from build123d import *

# Parameters (mm, degrees)
F0_W      = 19.9827682227
F0_H      = 13.8834062964
F2_R      = 5
F3_SIZE   = 5
F5_D      = 3
F7_D      = 3
F9_D      = 3
F11_DEPTH = 2


with BuildPart() as f1:
    # F0 (on Front) → F1 (revolve)
    with BuildSketch(Plane.XZ):
        Polygon((-5.1426226273, 40.0602705777), (-45.9897518158, 40.0602705777), (-45.9897518158, 11.2985512242), (-5.1426226273, 11.2985512242), (-5.1426226273, 26.1768642813), align=None)
        with Locations((4.848761484, 33.1185674295)):
            Rectangle(F0_W, F0_H)
    revolve(axis=Axis((-8.3751268685, 0, 0), (1, 0, 0)))

    # F2
    f2_edges = [f1.edges().sort_by_distance(p)[0] for p in [
        (14.840146, 0, -26.176864),
    ]]
    fillet(f2_edges, radius=F2_R)

    # F3
    f3_edges = [f1.edges().sort_by_distance(p)[0] for p in [
        (-5.142623, 0, -26.176864),
        (14.840146, 0, -40.060271),
        (-45.989752, 0, -40.060271),
        (-15.574803, 0, 40.060271),
    ]]
    chamfer(f3_edges, length=F3_SIZE)

    # F5 (through all)
    with Locations(Plane.YZ.offset(-5.1426226273)):
        with Locations((-16.2885512242, 0)):
            Hole(F5_D / 2)

    # F7 (through all)
    with Locations(Plane.YZ.offset(-5.1426226273)):
        with Locations((15.9020125866, 0)):
            Hole(F7_D / 2)

    # F9 (through all)
    with Locations(Plane.YZ.offset(-5.1426226273)):
        with Locations((0, 16.050176695)):
            Hole(F9_D / 2)

    # F10 (on face) → F11 (cut)
    with BuildSketch(Plane.YZ.offset(-5.1426226273)):
        with BuildLine():
            Line((5.9653543867, 17.550176695), (0, 17.550176695))
            ThreePointArc((0, 17.550176695), (1.0606601718, 17.1108368668), (1.5, 16.050176695))
            ThreePointArc((1.5, 16.050176695), (1.2449620199, 15.2134750941), (0.5665739081, 14.6612944081))
            Line((0.5665739081, 14.6612944081), (5.9653543867, 14.6612944081))
            Line((5.9653543867, 14.6612944081), (5.9653543867, 17.550176695))
        make_face()
    extrude(amount=-F11_DEPTH, mode=Mode.SUBTRACT)


solid = f1.part
Build history of the part. All positions in model axes, mm. A direction names the side the tool comes from. Round coordinates to 2 decimals unless told otherwise and drop trailing zeros. Write each loop counter-clockwise with the first axis right and the second up, starting at its lowest first coordinate (ties: lowest second). Pieces come first, ordered by that corner, then holes. Notation, with made-up numbers: M -35.5,6.5 L 21.5,6.5 A33 cw 21.5,34.5 Z; hole C 50.25,62 d5. An arc over 180 degrees is marked long. Use CSV: the item, a comma, the result in double quotes.
1. Two-plate mould, pull along Y, no slides. Class faces 1 (the face through (-25.85, -17.72, 0.45)), 2 (the face through (-6, 3, 14.661)), 3 (the face through (-45.747, 21.481, -28.015)), 4 (the face through (-45.99, -8.3, -8.3)): +Y half, -Y half, draft (parallel to the pull), parting line (faces both ways), or undercut.
Reply:
face 1,"undercut"
face 2,"undercut"
face 3,"parting line"
face 4,"draft"
2. Saw through at B-B (x = -33). Give the cut face in (y, z), plus the area to 3 significant figures.
Reply:
outline,"C 0,0 d80.12; hole C -16.29,0 d3; hole C 0,0 d22.6; hole C 0,16.05 d3; hole C 15.9,0 d3"
area,"4,620 mm²"
3. Wall check: probe 1 along Z at (x, y) = (-36, 0); probe 2 along Z at (x, y) = (-42, -10); probe 3 along Z at (x, y) = (-35, -16). Give the ranges that are in metal, low to high. Write a range as from..to.
Reply:
probe 1,"z = -40.06..-11.3, 11.3..14.55, 17.55..40.06"
probe 2,"z = -37.75..-5.26, 5.26..37.75"
probe 3,"z = -36.73..-1.47, 1.47..36.73"
4. Tool access for faces 5 (the face through (-25.28, 6.87, -8.97)), 6 (the face through (-6, 5.965, 16)): list every direction of +Z, -Z, +X, -X, +Y, -Y with a clear straight run to the whole face (end or side of a thin tool).
Reply:
face 5,"+X, -X"
face 6,"+X"
5. Saw through at A-A (z = 0). Give the cut face in (x, y).
Reply:
outline,"M -45.99,-35.06 L -40.99,-40.06 L 9.84,-40.06 L 14.84,-35.06 L 14.84,-31.18 A5 ccw 9.84,-26.18 L -0.14,-26.18 L -5.14,-21.18 L -5.14,-17.79 L -45.99,-17.79 Z; M -45.99,-14.79 L -5.14,-14.79 L -5.14,-11.3 L -45.99,-11.3 Z; M -45.99,11.3 L -5.14,11.3 L -5.14,14.4 L -45.99,14.4 Z; M -45.99,17.4 L -5.14,17.4 L -5.14,21.18 L -0.14,26.18 L 9.84,26.18 A5 ccw 14.84,31.18 L 14.84,35.06 L 9.84,40.06 L -40.99,40.06 L -45.99,35.06 Z"
6. Flat gauge pins, fed straight in: pin 1 (0.6 mm diameter, centred on x = -6.5, y = 4, fed in from +Z); pin 2 (2 mm diameter, centred on x = -36, y = -23, fed in from +Z); pin 3 (1 mm diameter, centred on y = 6, z = -26.5, fed in from +X); pin 4 (1.8 mm diameter, centred on y = 15.9, z = 0, fed in from +X). Where does each tip first touch, or does it go through?
Reply:
pin 1,"stops at z = 39.89"
pin 2,"stops at z = 33.48"
pin 3,"stops at x = 13.4"
pin 4,"passes through"
7. Saw through at C-C (x = 5.5). Give the cut face in (y, z).
Reply:
outline,"C 0,0 d80.12; hole C 0,0 d52.35"
